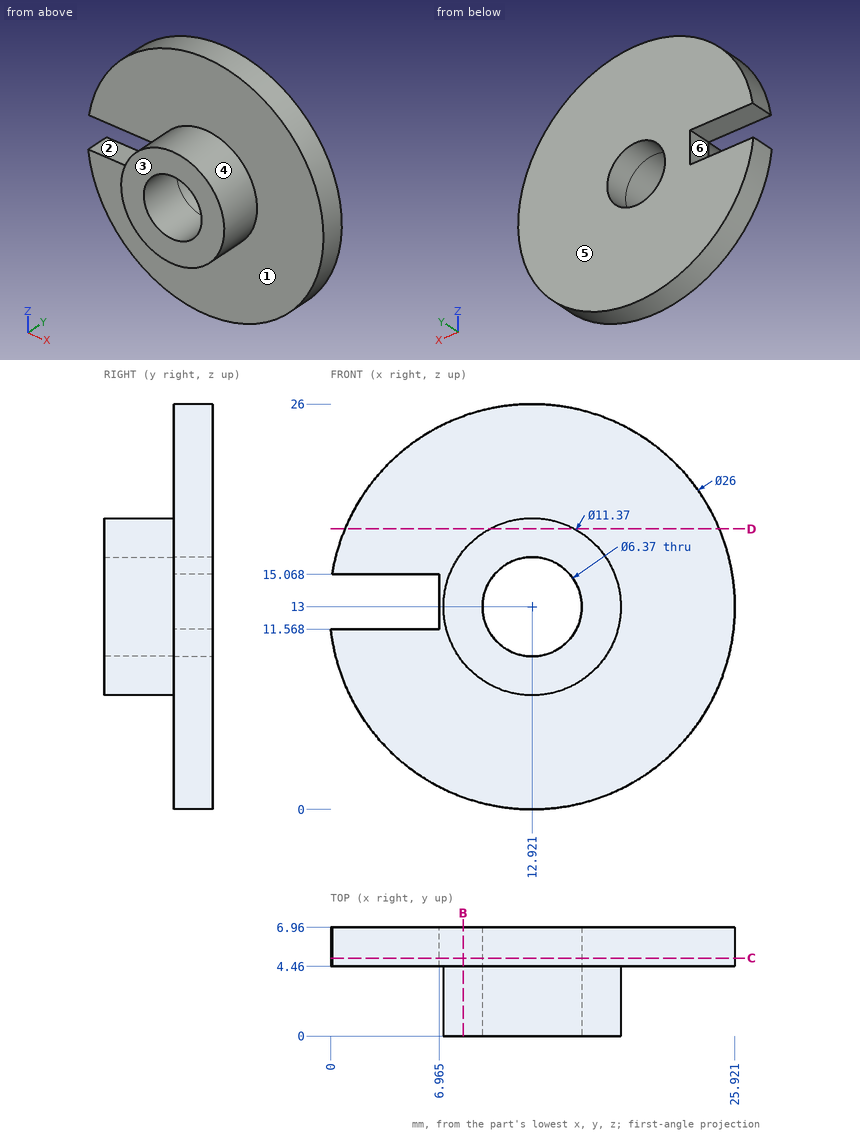
Study the drawing (mm; zero at the part's minimum x, y, z) and answer. A direction names the side the tool comes from. Coordinates: 2 decimals unless noted, no trailing zeros. Write each loop counter-clockwise with the first axis right and the second up, starting at its lowest first coordinate (ties: lowest second). Pieces come first, ordered by that corner, then holes. Notation, with made-up numbers: (24, 39.5) - (32, 39.5) arc R21 cw to (32, 55.5) - close; hole circle Ø10 at (37, -30). An arc over 180 degrees is marked (long way). One line per question, with ' | ' between items.
1) The mould has two halves that part along Z. Classify the marked faces 4, 5 and 6: +Z half, -Z half, draft (parallel to the pull), parting line (faces both ways), or undercut.
Checks:
face 4: parting line | face 5: draft | face 6: undercut
2) For the marked faces 1, 2 and 3, determine the directions among +Z, -Z, +X, -X, +Y, -Y from which every point of the face is accessible in a straight line to the end or side of a thin tool.
Checks:
face 1: -Y | face 2: -X, +Y, -Y | face 3: +Z, -Z, +X, -X, -Y
3) Find section B-B, the plane x = 8.5. Determine the outline of the cut face in (y, z) (1 decimal).
Checks:
outline: (0, 9.4) - (4.5, 9.4) - (4.5, 0.8) - (7, 0.8) - (7, 25.2) - (4.5, 25.2) - (4.5, 16.6) - (0, 16.6) - close
4) Consider probe 1 along X at (y, z) = (2.6, 13); probe 2 along Z at (x, y) = (13.75, 2) (1 decimal); probe 3 along Y at (x, z) = (11.25, 22.5). Determine where each line is inside the solid, lowest interval first. Write a range as [from, to].
Checks:
probe 1: [7.24, 9.74], [16.11, 18.61] | probe 2: [7.4, 9.9], [16.1, 18.6] | probe 3: [4.46, 6.96]
5) Find section D-D, the plane z = 18. Determine the outline of the cut face in (x, y) (1 decimal).
Checks:
outline: (0.9, 4.5) - (10.2, 4.5) - (10.2, 0) - (15.6, 0) - (15.6, 4.5) - (24.9, 4.5) - (24.9, 7) - (0.9, 7) - close
6) Flat-ended cylindrical pins translate along their axes: P1, Ø1.5, axis at x = 20.5, z = 22, coming from the -Y side; P2, Ø2, axis at x = 2, y = 6, coming from the +Z side; P3, Ø1.2, axis at x = 3.5, y = 6.5, coming from the -Z side. Find the tip coordinate at first contact, or state that the pin passes through.
Checks:
P1: y = 4.46 | P2: z = 21.4 | P3: z = 3.45
7) Find section C-C, the plane y = 5. Determine the outline of the cut face in (x, z) (1 decimal).
Checks:
outline: (0, 11.6) arc R13 ccw (long way) to (0.1, 15.1) - (7, 15.1) - (7, 11.6) - close; hole circle Ø6.4 at (12.9, 13)
